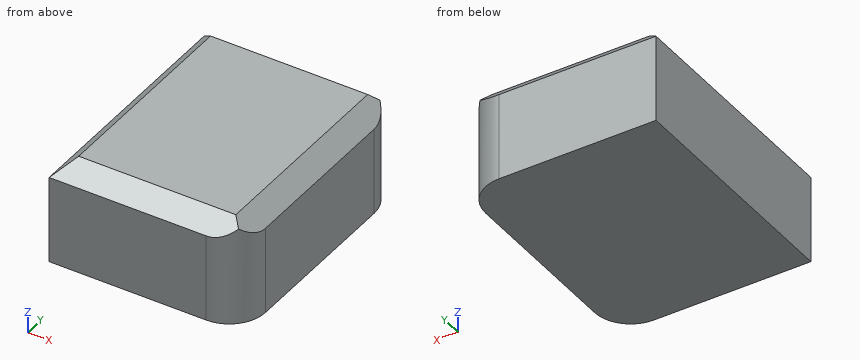
from build123d import *

# Parameters (mm, degrees)
F0_W     = 39.1064089628
F0_H     = 16.67773308
F1_DEPTH = 68.1895
F2_SIZE2 = 5.08
F2_SIZE  = 5.08
F3_R     = 10.16


with BuildPart() as f1:
    # F0 (on Front) → F1 (new body)
    with BuildSketch(Plane.XZ):
        with Locations((34.7932044814, 21.27848872)):
            Rectangle(F0_W, F0_H)
        Polygon((0, 29.6173552599), (0, 0), (54.3464089628, 0), (54.3464089628, 12.93962218), (15.24, 12.93962218), (15.24, 29.6173552599), align=None)
    extrude(amount=F1_DEPTH)

    # F2
    f2_edges = [f1.edges().sort_by_distance(p)[0] for p in [
        (54.346409, -34.09475, 29.617355),
        (27.173204, 0, 29.617355),
        (0, -34.09475, 29.617355),
        (27.173204, -68.1895, 29.617355),
    ]]
    chamfer(f2_edges, length=F2_SIZE, length2=F2_SIZE2)

    # F3
    f3_edges = [f1.edges().sort_by_distance(p)[0] for p in [
        (54.346409, 0, 12.268678),
        (54.346409, -68.1895, 12.268678),
    ]]
    fillet(f3_edges, radius=F3_R)


solid = f1.part
The listing builds one solid part. Answer for the finished solid, in the listing's coordinates (mm). Give positions to 0.01 mm unless a question says otherwise; leave off trailing zeros. Loops run counter-clockwise (first coordinate to the right, second up) from the corner with the lowest first, then second, coordinate; pieces in that order, holes last. Notation, with made-up numbers: (-30, 60.5) - (-1, 60.5) arc R9 cw to (-1, 71.5) - close; hole circle Ø1 at (1.25, -30.75). An arc over 180 degrees is marked (long way). Write each question's results on one line, items separated by ' | '.
1. Find section B-B, the plane z = 26.75. Write down the section's boundary in (x, y).
Resolved:
outline: (2.21, -65.98) - (50.52, -65.98) arc R10.16 ccw to (52.13, -64.36) - (52.13, -3.83) arc R10.16 ccw to (50.52, -2.21) - (2.21, -2.21) - close
2. Consider probe 1 along Y at (x, z) = (50, 4); probe 2 along Y at (x, z) = (48.5, 15); probe 3 along X at (y, z) = (-61.5, 12.25). Determine where each line is inside the solid, lowest interval first. Write a range as from..to.
Resolved:
probe 1: y = -66.36..-1.83 | probe 2: y = -67.23..-0.96 | probe 3: x = 0..53.74
3. Find section A-A, the plane y = -16.5. Write down the section's boundary in (x, z), then the cut area to 3 significant figures.
Resolved:
outline: (0, 0) - (54.35, 0) - (54.35, 24.54) - (49.27, 29.62) - (5.08, 29.62) - (0, 24.54) - close | area: 1,580 mm^2
